For this review, take the finished solid that the model builds, in its own axes (mm). A direction names the side the tool comes from. Round coordinates to 2 decimals unless told otherwise and drop trailing zeros. Write each loop counter-clockwise with the first axis right and the second up, starting at its lowest first coordinate (ties: lowest second). Pieces come first, ordered by that corner, then holes. Notation, with made-up numbers: (58, 40) -> (82, 40) arc R20 cw to (82, 70) -> close; hole circle Ø7 at (-4.75, 31.5). An arc over 180 degrees is marked (long way). Answer in a Markdown table with one row per item.
from build123d import *

# Parameters (mm, degrees)
SKETCH_1_W          = 55
SKETCH_1_H          = 30
EXTRUDE_1_DEPTH     = 19
SKETCH_2_R          = 2.4
CUT_EXTRUDE_1_DEPTH = 37.636730203
SKETCH_3_W          = 10
SKETCH_3_H          = 14
CUT_EXTRUDE_2_DEPTH = 5


with BuildPart() as part:
    # 草图1 → 凸台-拉伸1 (new body)
    with BuildSketch(Plane(origin=(0, 0, 0), x_dir=(1, 0, 0), z_dir=(0, 1, 0))):
        Rectangle(SKETCH_1_W, SKETCH_1_H)
    extrude(amount=EXTRUDE_1_DEPTH)

    # 草图2 → 切除-拉伸1 (cut, through all)
    with BuildSketch(Plane(origin=(0, 19, 0), x_dir=(1, 0, 0), z_dir=(0, 1, 0))):
        with Locations(Location((-22, 0, 0), (0, 0, 270))):
            Circle(SKETCH_2_R)
        with Locations(Location((22, 0, 0), (0, 0, 90))):
            Circle(SKETCH_2_R)
    extrude(amount=-CUT_EXTRUDE_1_DEPTH, mode=Mode.SUBTRACT)

    # 草图3 → 切除-拉伸2 (cut)
    with BuildSketch(Plane(origin=(0, 19, 0), x_dir=(1, 0, 0), z_dir=(0, 1, 0))):
        with Locations((-12, 8)):
            Rectangle(SKETCH_3_W, SKETCH_3_H)
        with Locations((0, 8)):
            Rectangle(SKETCH_3_W, SKETCH_3_H)
        with Locations((12, 8)):
            Rectangle(SKETCH_3_W, SKETCH_3_H)
        with Locations((12, -8)):
            Rectangle(SKETCH_3_W, SKETCH_3_H)
        with Locations((0, -8)):
            Rectangle(SKETCH_3_W, SKETCH_3_H)
        with Locations((-12, -8)):
            Rectangle(SKETCH_3_W, SKETCH_3_H)
    extrude(amount=-CUT_EXTRUDE_2_DEPTH, mode=Mode.SUBTRACT)


solid = part.part
1) Consider section B-B on z = 0. State the section outline as (x, y) points, then the cut area to 3 significant figures.
Solved:
| item | result |
|---|---|
| outline | (-27.5, 0) -> (-24.4, 0) -> (-24.4, 19) -> (-27.5, 19) -> close; (-19.6, 0) -> (19.6, 0) -> (19.6, 19) -> (-19.6, 19) -> close; (24.4, 0) -> (27.5, 0) -> (27.5, 19) -> (24.4, 19) -> close |
| area | 863 mm² |
2) Consider section C-C on y = 3.5. State the section outline as (x, z) points.
Solved:
| item | result |
|---|---|
| outline | (-27.5, -15) -> (27.5, -15) -> (27.5, 15) -> (-27.5, 15) -> close; hole circle Ø4.8 at (-22, 0); hole circle Ø4.8 at (22, 0) |
3) For faces 1 (the flat face through (0, 9, -15)), 2 (the flat face through (-12, 17, 1)), 3 (the flat face through (17, 17, -8)), list the 3-axis set-ups (+Z, -Z, +X, -X, +Y, -Y) from which the entire face can be reached by the end or side of a thin tool; tool diameter is ignored.
Solved:
| item | result |
|---|---|
| face 1 | -Z, +X, -X, +Y, -Y |
| face 2 | +Z, +Y |
| face 3 | -Z, +Y |
4) Mouldability with a two-part tool opening along X and no side actions: class faces 4 (the flat face through (-27.5, 9, 0)), 5 (the flat face through (27.5, 9, 0)), 6 (the flat face through (-7, 17, -8)), 7 (the flat face through (5, 17, -8)) as pulls with the +X half, pulls with the -X half, needs draft (parallel to the pull), parting line crosses it, or undercut.
Solved:
| item | result |
|---|---|
| face 4 | pulls with the -X half |
| face 5 | pulls with the +X half |
| face 6 | undercut |
| face 7 | undercut |
5) Clearance check with flat-ended pins moving along their axes: pin 1 Ø4 at (x, y) = (-10, 17.5) entering from +Z; pin 2 Ø1.5 at (x, y) = (13, 15.5) entering from -Z; pin 3 Ø5 at (x, z) = (1, -7.5) entering from +Y. State where each tip first meets the part, or that it passes through.
Solved:
| item | result |
|---|---|
| pin 1 | z = 1 |
| pin 2 | z = -1 |
| pin 3 | y = 14 |
6) Consider section A-A on x = 22. State the section outline as (y, z) points.
Solved:
| item | result |
|---|---|
| outline | (0, -15) -> (19, -15) -> (19, -2.4) -> (0, -2.4) -> close; (0, 2.4) -> (19, 2.4) -> (19, 15) -> (0, 15) -> close |
7) For line 1 (X direction, y = 17.5, z = 11); line 2 (X direction, y = 6.25, z = 0.5); line 3 (Z direction, x = 22, y = 11.75), list the stretches that pass through material, from the lowest coordinate up. Write a range as [from, to].
Solved:
| item | result |
|---|---|
| line 1 | [-27.5, -17], [-7, -5], [5, 7], [17, 27.5] |
| line 2 | [-27.5, -24.35], [-19.65, 19.65], [24.35, 27.5] |
| line 3 | [-15, -2.4], [2.4, 15] |
8) Consider section D-D on z = -3.75. State the section outline as (x, y) points.
Solved:
| item | result |
|---|---|
| outline | (-27.5, 0) -> (27.5, 0) -> (27.5, 19) -> (17, 19) -> (17, 14) -> (7, 14) -> (7, 19) -> (5, 19) -> (5, 14) -> (-5, 14) -> (-5, 19) -> (-7, 19) -> (-7, 14) -> (-17, 14) -> (-17, 19) -> (-27.5, 19) -> close |
